from build123d import *

# Parameters (mm, degrees)
SKETCH2_R                = 2.5
BOSS_EXTRUDE1_DEPTH      = 35.494976
BOSS_EXTRUDE1_DEPTH_BACK = 35.494976
SKETCH3_R                = 3.175
BOSS_EXTRUDE2_DEPTH      = 20.32
BOSS_EXTRUDE2_DEPTH_BACK = 20.32


with BuildPart() as part:
    # Sketch2 → Boss-Extrude1 (new body, two sides)
    with BuildSketch(Plane.XY) as boss_extrude1_sk:
        Circle(SKETCH2_R)
    extrude(amount=BOSS_EXTRUDE1_DEPTH)
    extrude(boss_extrude1_sk.sketch, amount=-BOSS_EXTRUDE1_DEPTH_BACK)

    # Sketch3 → Boss-Extrude2 (add, two sides)
    with BuildSketch(Plane.XY) as boss_extrude2_sk:
        Circle(SKETCH3_R)
    extrude(amount=BOSS_EXTRUDE2_DEPTH)
    extrude(boss_extrude2_sk.sketch, amount=-BOSS_EXTRUDE2_DEPTH_BACK)


solid = part.part
Geometry: final body of the model. Coordinates: model frame, mm. A direction names the side the tool comes from. Round coordinates to 2 decimals unless told otherwise and drop trailing zeros. Order: outer loops, then holes, each group sorted by start corner. A loop starts at its lowest first (then second) coordinate and runs counter-clockwise, first axis right, second up. Notation, with made-up numbers: (-17.5, 58) - (37.5, 58) arc R19 cw to (37.5, 67) - close; hole circle Ø6 at (51.25, 80). An arc over 180 degrees is marked (long way). Write each question's results on one line, items separated by ' | '.
Item 1: First-contact query: pin 1 Ø1.5 at (x, z) = (-1, 27) entering from +Y; pin 2 Ø3 at (y, z) = (-2, 3) entering from +X. Flat tips, straight axial feed; report the tip coordinate or a pass-through.
Completed:
pin 1: y = 2.49 | pin 2: x = 3.14
Item 2: Section A-A, the plane y = 0. Return the cut outline in (x, z) (3 decimals), and give its area (3 significant figures).
Completed:
outline: (-3.175, -20.32) - (-2.5, -20.32) - (-2.5, -35.495) - (2.5, -35.495) - (2.5, -20.32) - (3.175, -20.32) - (3.175, 20.32) - (2.5, 20.32) - (2.5, 35.495) - (-2.5, 35.495) - (-2.5, 20.32) - (-3.175, 20.32) - close | area: 410 mm^2
Item 3: Section C-C, the plane z = 8.5. Return the cut outline in (x, y) (3 decimals).
Completed:
outline: circle Ø6.35 at (0, 0)
Item 4: Reachability of faces 1 (the flat face through (0, -3, 20.32)), 2 (the cylindrical face through (-0.54, -2.44, -27.8)), 3 (the cylindrical face through (-0.69, -3.1, 0.28)) from +Z, -Z, +X, -X, +Y, -Y: full face, straight path, thin tool, end or side. Return the list, or none.
Completed:
face 1: +Z | face 2: -Z | face 3: +Z, -Z
Item 5: Section D-D, the plane z = 29. Return the cut outline in (x, y), and give its area (3 significant figures).
Completed:
outline: circle Ø5 at (0, 0) | area: 19.6 mm^2
Item 6: Material intervals for line 1 along Z through (x, y) = (1.25, -2.5); line 2 along Y through (x, z) = (1, -18.5); line 3 along X through (y, z) = (-2.5, 19), sorted ascending. Write a range as [from, to].
Completed:
line 1: [-20.32, 20.32] | line 2: [-3.01, 3.01] | line 3: [-1.96, 1.96]
